Check sheet for the modelled part. Datum: model origin and axes. Units: mm. Face numbers are marked on the shaded views. Round coordinates to 2 decimals unless told otherwise and drop trailing zeros. Write each loop counter-clockwise with the first axis right and the second up, starting at its lowest first coordinate (ties: lowest second). Pieces come first, ordered by that corner, then holes.
Item 1: Cross-section at A-A on x = 31. Enter the section's corners in (y, z).
Item 2: Material ranges on line 1 (X direction, y = 1.1, z = -7.5); line 2 (Z direction, x = 5.5, y = 1.6); line 3 (Z direction, x = 12, y = 7.75), recorded low to high.
Item 3: Release check for a two-part mould opening along X. For the marked faces 1, 2, 3 and 4 record: +X half, -X half, draft (parallel to the pull), parting line (faces both ways), or undercut.
Item 4: Cross-section at C-C on y = 19. Enter the section's corners in (x, z).
Item 5: Cross-section at B-B on y = 8. Enter the section's corners in (x, z), plus the area to 3 significant figures.
Item 6: Cross-section at D-D on x = 40. Enter the section's corners in (y, z), plus the area to 4 significant figures.
Item 7: Go/stop test with a flat-tipped pin: pin 1 Ø1.2 at (x, z) = (53, -21) entering from +Y. Record where the tip stops, or that it passes through.
from build123d import *

# Parameters (mm, degrees)
SKETCH1_W                      = 62
SKETCH1_H                      = 28
BOSS_EXTRUDE1_DEPTH            = 25
SKETCH2_W                      = 58
SKETCH2_H                      = 24
CUT_EXTRUDE1_DEPTH             = 23
BOSS_EXTRUDE3_DEPTH            = 58
F_1_5_1_5_DIAMETER_HOLE1_D     = 1.5
F_2_0_2_DIAMETER_HOLE1_D       = 2
F_2_0_2_DIAMETER_HOLE1_DEPTH   = 2
F_3_5_3_5_DIAMETER_HOLE1_D     = 3.5
F_3_5_3_5_DIAMETER_HOLE1_DEPTH = 2
BOSS_EXTRUDE4_REACH            = 72.774
F_3_0_3_DIAMETER_HOLE1_REACH   = 73.197
F_3_0_3_DIAMETER_HOLE1_BORE_R  = 1.5


with BuildPart() as part:
    # Sketch1 → Boss-Extrude1 (new body)
    with BuildSketch(Plane(origin=(0, 0, 0), x_dir=(1, 0, 0), z_dir=(0, 1, 0))):
        with Locations((31, 14)):
            Rectangle(SKETCH1_W, SKETCH1_H)
    extrude(amount=BOSS_EXTRUDE1_DEPTH)

    # Sketch2 → Cut-Extrude1 (cut)
    with BuildSketch(Plane(origin=(0, 25, 0), x_dir=(1, 0, 0), z_dir=(0, 1, 0))):
        with Locations((31, 14)):
            Rectangle(SKETCH2_W, SKETCH2_H)
    extrude(amount=-CUT_EXTRUDE1_DEPTH, mode=Mode.SUBTRACT)

    # Sketch3 → Boss-Extrude3 (add)
    with BuildSketch(Plane(origin=(2, 0, 0), x_dir=(0, 0, -1), z_dir=(1, 0, 0))):
        Polygon((26, 11), (21, 21), (26, 21), align=None)
    extrude(amount=BOSS_EXTRUDE3_DEPTH)

    # Ø1.5 (1.5) Diameter Hole1 (through all)
    with Locations(Plane(origin=(0, 0, 0), x_dir=(-1, 0, 0), z_dir=(0, -1, 0))):
        with Locations((-7.5, 7.5), (-5.5, 7.5), (-3.5, 7.5)):
            Hole(F_1_5_1_5_DIAMETER_HOLE1_D / 2)

    # Ø2.0 (2) Diameter Hole1
    with Locations(Plane(origin=(0, 0, 0), x_dir=(-1, 0, 0), z_dir=(0, -1, 0))):
        with Locations((-53, 21)):
            Hole(F_2_0_2_DIAMETER_HOLE1_D / 2, depth=F_2_0_2_DIAMETER_HOLE1_DEPTH)

    # Ø3.5 (3.5) Diameter Hole1
    with Locations(Plane(origin=(0, 0, 0), x_dir=(-1, 0, 0), z_dir=(0, -1, 0))):
        with Locations((-40, 22)):
            Hole(F_3_5_3_5_DIAMETER_HOLE1_D / 2, depth=F_3_5_3_5_DIAMETER_HOLE1_DEPTH)

    # Sketch10 → Boss-Extrude4 (add, up to next)
    with BuildSketch(Plane(origin=(2, 0, 0), x_dir=(0, 0, -1), z_dir=(1, 0, 0)), mode=Mode.PRIVATE) as boss_extrude4_sk1:
        Polygon((26, 4), (23, 7), (26, 7), align=None)
    boss_extrude4_tool1 = extrude(boss_extrude4_sk1.sketch, amount=BOSS_EXTRUDE4_REACH, mode=Mode.PRIVATE) - part.part
    add(boss_extrude4_tool1.solids().sort_by_distance((2, 6, -25))[0])

    # Ø3.0 (3) Diameter Hole1 bore → Ø3.0 (3) Diameter Hole1 (cut, up to next)
    with BuildSketch(Plane(origin=(0, 21, 0), x_dir=(1, 0, 0), z_dir=(0, 1, 0)), mode=Mode.PRIVATE) as f_3_0_3_diameter_hole1_sk1:
        with Locations((31, 23.5)):
            Circle(F_3_0_3_DIAMETER_HOLE1_BORE_R)
    f_3_0_3_diameter_hole1_tool1 = extrude(f_3_0_3_diameter_hole1_sk1.sketch, amount=-F_3_0_3_DIAMETER_HOLE1_REACH, mode=Mode.PRIVATE) & part.part
    add(f_3_0_3_diameter_hole1_tool1.solids().sort_by_distance((31, 21, -23.5))[0], mode=Mode.SUBTRACT)


solid = part.part
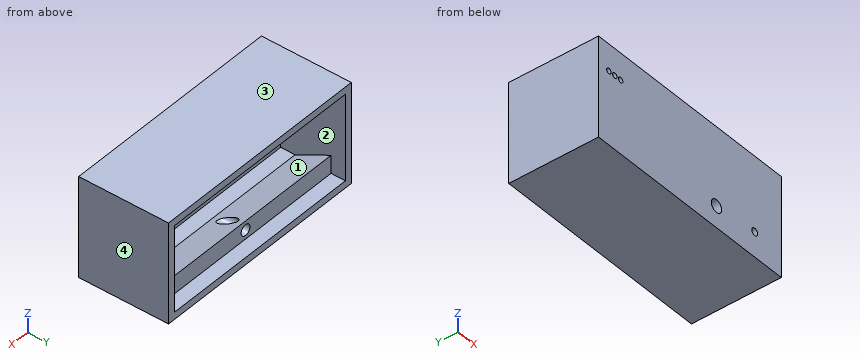
Response values:
1. outline: (0, -28) - (25, -28) - (25, -26) - (21, -26) - (21, -25) - (13, -25) - (11, -26) - (7, -26) - (7, -23) - (4, -26) - (2, -26) - (2, -2) - (25, -2) - (25, 0) - (0, 0) - close; (19, -22) - (21, -22) - (21, -21) - close
2. line 1: x = 0 to 2.75, 4.25 to 4.75, 6.25 to 6.75, 8.25 to 62
2. line 2: z = -28 to -8.25, -6.75 to 0
2. line 3: z = -28 to -26, -2 to 0
3. face 1: undercut
3. face 2: undercut
3. face 3: draft
3. face 4: +X half
4. outline: (0, -28) - (62, -28) - (62, 0) - (0, 0) - close; hole (2, -22) - (60, -22) - (60, -2) - (2, -2) - close; hole circle Ø3 at (31, -23.5)
5. outline: (0, -28) - (62, -28) - (62, 0) - (0, 0) - close; hole (2, -26) - (60, -26) - (60, -2) - (2, -2) - close
5. area: 344 mm2
6. outline: (0, -28) - (25, -28) - (25, -26) - (21, -26) - (21, -21) - (11, -26) - (7, -26) - (7, -23) - (4, -26) - (2, -26) - (2, -23.75) - (0, -23.75) - close; (0, -20.25) - (2, -20.25) - (2, -2) - (25, -2) - (25, 0) - (0, 0) - close
6. area: 170.5 mm2
7. pin 1: stops at y = 21
